from build123d import *

# Parameters (mm, degrees)
SKETCH1_R           = 2
BOSS_EXTRUDE1_DEPTH = 29.5
CHAMFER1_SIZE       = 0.5
CUT_EXTRUDE1_DEPTH  = 2


with BuildPart() as part:
    # Sketch1 → Boss-Extrude1 (new body)
    with BuildSketch(Plane(origin=(0, 0, 0), x_dir=(1, 0, 0), z_dir=(0, 1, 0))):
        Circle(SKETCH1_R)
    extrude(amount=BOSS_EXTRUDE1_DEPTH)

    # Chamfer1
    chamfer1_edges = [part.edges().sort_by_distance(p)[0] for p in [
        (-2, 0, 0),
    ]]
    chamfer(chamfer1_edges, length=CHAMFER1_SIZE)

    # Sketch2 → Cut-Extrude1 (cut)
    with BuildSketch(Plane(origin=(0, 29.5, 0), x_dir=(1, 0, 0), z_dir=(0, 1, 0))):
        Polygon((1.1, 0.635085296), (0, 1.270170592), (-1.1, 0.635085296), (-1.1, -0.635085296), (0, -1.270170592), (1.1, -0.635085296), align=None)
    extrude(amount=-CUT_EXTRUDE1_DEPTH, mode=Mode.SUBTRACT)


solid = part.part
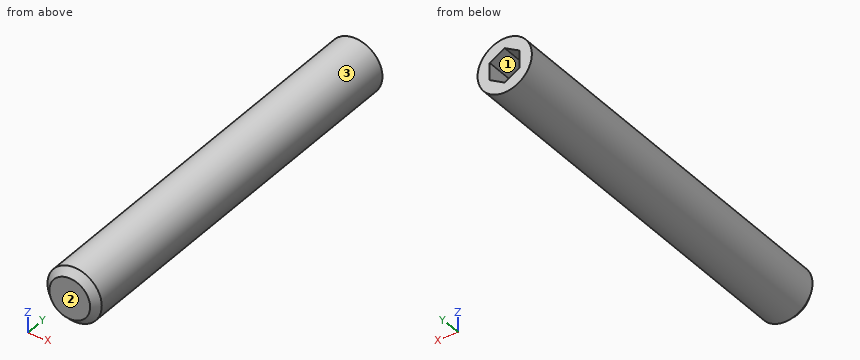
Read the model definition and answer for the solid it produces. Units are mm, in the model's axes. Face numbers are marked on the shaded views. Give positions to 0.01 mm unless a question says otherwise; leave off trailing zeros. Write each loop counter-clockwise with the first axis right and the second up, starting at its lowest first coordinate (ties: lowest second). Pieces come first, ordered by that corner, then holes. Notation, with made-up numbers: (80, 27.25) -> (112, 27.25) arc R15 ccw to (112, 36.25) -> close; hole circle Ø1 at (52, -37.75). An arc over 180 degrees is marked (long way). Answer as a JSON object with one key per item and string values. Group by question number.
1) Find section B-B (y = 10). Write down the section's boundary in (x, z).
2) This flat-tipped pin is pushed along its axis until it touches: P1, Ø0.7, axis at x = 0, z = 0.5, coming from the +Y side. Where does it stop, or does it pass through?
3) Find section A-A (z = 0). Write down the section's boundary in (x, y).
4) Consider L1, parallel to Z at x = -0.1, y = 17; L2, parallel to Z at x = 1.55, y = 19.75. Determine where each line is inside the solid, lowest interval first. Write a range as from..to.
5) The mould has two halves that part along X. Classify the marked faces 1, 2 and 3: +X half, -X half, draft (parallel to the pull), parting line (faces both ways), or undercut.
Values follow:
{
 "1": {"outline": "circle Ø4 at (0, 0)"},
 "2": {"P1": "stops at y = 27.5"},
 "3": {"outline": "(-2, 0.5) -> (-1.5, 0) -> (1.5, 0) -> (2, 0.5) -> (2, 29.5) -> (1.1, 29.5) -> (1.1, 27.5) -> (-1.1, 27.5) -> (-1.1, 29.5) -> (-2, 29.5) -> close"},
 "4": {"L1": "z = -2..2", "L2": "z = -1.26..1.26"},
 "5": {"face 1": "undercut", "face 2": "draft", "face 3": "parting line"}
}
